from build123d import *

# Parameters (mm, degrees)
SKETCH1_W           = 40
SKETCH1_H           = 15
BOSS_EXTRUDE1_DEPTH = 1000
SKETCH2_W           = 5
SKETCH2_H           = 60
BOSS_EXTRUDE2_DEPTH = 100


with BuildPart() as part:
    # Sketch1 → Boss-Extrude1 (new body)
    with BuildSketch(Plane(origin=(0, 0, 0), x_dir=(0, 0, -1), z_dir=(1, 0, 0))):
        Polygon((50, -7.5), (20, -7.5), (-20, -7.5), (-50, -7.5), (-50, -22.5), (50, -22.5), align=None)
        Rectangle(SKETCH1_W, SKETCH1_H)
    extrude(amount=-BOSS_EXTRUDE1_DEPTH)

    # Sketch2 → Boss-Extrude2 (add)
    with BuildSketch(Plane.XY.offset(50)):
        with Locations((-2.5, 7.5)):
            Rectangle(SKETCH2_W, SKETCH2_H)
    boss_extrude2 = extrude(amount=-BOSS_EXTRUDE2_DEPTH)

    # Mirror1: Boss-Extrude2 across plane
    add(boss_extrude2.mirror(Plane.ZY.offset(500)))


solid = part.part
The model under review builds one solid part; all positions refer to its coordinate system, in mm. A direction names the side the tool comes from. Round coordinates to 2 decimals unless told otherwise and drop trailing zeros. Order: outer loops, then holes, each group sorted by start corner. A loop starts at its lowest first (then second) coordinate and runs counter-clockwise, first axis right, second up. Notation, with made-up numbers: (49.25, 19) -> (75.25, 19) arc R17 cw to (75.25, 48) -> close; hole circle Ø10 at (56, 87.5). An arc over 180 degrees is marked (long way). Return JSON: item names as keys, results as strings.
1. The part is to be moulded in two halves that separate along X. For faces 6 (the face through (-493, -7.5, -35)), 7 (the face through (-498, -17, -50)), 8 (the face through (-1000, 8, 1)), say which applies: +X half, -X half, draft (parallel to the pull), parting line (faces both ways), or undercut.
Answer block:
{"face 6": "undercut", "face 7": "draft", "face 8": "-X half"}
2. Insertion check: P1, Ø15, axis at x = -675, z = 36, coming from the +Y side; P2, Ø12, axis at x = -199, y = 4, coming from the +Z side; P3, Ø10, axis at x = -304.5, y = -5.5, coming from the -Z side; P4, Ø20, axis at x = -686, z = 1.5, coming from the +Y side. Each pin has a flat end and moves straight along its axis. Give the tip position at first contact, or say it passes through.
Answer block:
{"P1": "stops at y = -7.5", "P2": "stops at z = 20", "P3": "stops at z = -50", "P4": "stops at y = 7.5"}
3. Take a section at C-C (z = 1.5). Write out the cut boundary in (x, y).
Answer block:
{"outline": "(-1000, -22.5) -> (0, -22.5) -> (0, 37.5) -> (-5, 37.5) -> (-5, 7.5) -> (-995, 7.5) -> (-995, 37.5) -> (-1000, 37.5) -> close"}
4. For L1, parallel to X at y = 24.5, z = 10; L2, parallel to Z at x = -454, y = -6.5; L3, parallel to Y at x = -615.5, z = 13.5, list the stretches that pass through material, from the lowest coordinate up. Write a range as [from, to].
Answer block:
{"L1": "x = [-1000, -995], [-5, 0]", "L2": "z = [-20, 20]", "L3": "y = [-22.5, 7.5]"}
5. Take a section at A-A (y = 24). Write out the cut boundary in (x, z).
Answer block:
{"outline": "(-1000, -50) -> (-995, -50) -> (-995, 50) -> (-1000, 50) -> close; (-5, -50) -> (0, -50) -> (0, 50) -> (-5, 50) -> close"}
6. For faces 1 (the face through (-493, -22.5, 1)), 2 (the face through (-498, -12, 50)), 3 (the face through (-995, 15, 1)), 4 (the face through (-493, 7.5, 0)), 5 (the face through (-493, -7.5, 35)), list the 3-axis set-ups (+Z, -Z, +X, -X, +Y, -Y) from which the entire face can be reached by the end or side of a thin tool; tool diameter is ignored.
Answer block:
{"face 1": "+Z, -Z, +X, -X, -Y", "face 2": "+Z, +X, -X, +Y, -Y", "face 3": "+Y", "face 4": "+Z, -Z, +Y", "face 5": "+Z, +Y"}
7. Take a section at B-B (x = -82). Write out the cut boundary in (y, z), then the cut area to 3 significant figures.
Answer block:
{"outline": "(-22.5, -50) -> (-7.5, -50) -> (-7.5, -20) -> (7.5, -20) -> (7.5, 20) -> (-7.5, 20) -> (-7.5, 50) -> (-22.5, 50) -> close", "area": "2,100 mm²"}
